The listing builds one solid part. Answer for the finished solid, in the listing's coordinates (mm). A direction names the side the tool comes from. Give positions to 0.01 mm unless a question says otherwise; leave off trailing zeros. Order: outer loops, then holes, each group sorted by start corner. A loop starts at its lowest first (then second) coordinate and runs counter-clockwise, first axis right, second up.
```python
from build123d import *

# Parameters (mm, degrees)
F1_DEPTH = 40
F2_R     = 5


with BuildPart() as f1:
    # F0 (on Front) → F1 (new body)
    with BuildSketch(Plane.XZ):
        Polygon((30, 0), (0, 0), (-20, 10), (-20, 30), (-30, 30), (-30, -10), (30, -10), align=None)
    extrude(amount=F1_DEPTH)

    # F2
    f2_edges = [f1.edges().sort_by_distance(p)[0] for p in [
        (30, -40, -5),
        (30, 0, -5),
        (-25, -40, 30),
        (-25, 0, 30),
    ]]
    fillet(f2_edges, radius=F2_R)


solid = f1.part
```
1) A tool of negligible diameter and unlimited length cuts with its end or side. For faces 1 (the flat face through (30, -20, -5)), 2 (the flat face through (15, -20, 0)), from which of +Z, -Z, +X, -X, +Y, -Y can it reach the whole face along a straight path? Write none if from no direction.
Geometry says:
face 1: +Z, -Z, +X, +Y, -Y
face 2: +Z, +X, +Y, -Y
2) Given P1, Ø3, axis at y = -6.5, z = 8, coming from the +X side; P2, Ø1, axis at y = -17.5, z = 24.5, coming from the +X side; P3, Ø9, axis at x = 14, y = -26.5, coming from the +Z side, each flat-ended and moving along its own axis, determine where each tip first touches the part or whether it passes through.
Geometry says:
P1: stops at x = -13
P2: stops at x = -20
P3: stops at z = 0
3) Find section B-B (x = -12). Write down the section's boundary in (y, z), then the cut area to 3 significant figures.
Geometry says:
outline: (-40, -10) - (0, -10) - (0, 6) - (-40, 6) - close
area: 640 mm2
4) Find section C-C (z = 6). Write down the section's boundary in (x, y), then the cut area to 3 significant figures.
Geometry says:
outline: (-30, -40) - (-12, -40) - (-12, 0) - (-30, 0) - close
area: 720 mm2
5) Straight lines are drawn through the part: probe 1 along X at (y, z) = (-7, 21); probe 2 along Z at (x, y) = (19, -3); probe 3 along Z at (x, y) = (-8.5, -15.5). For each, find the intervals that lie inside material, in ascending order.
Geometry says:
probe 1: x = -30 to -20
probe 2: z = -10 to 0
probe 3: z = -10 to 4.25
6) Find section A-A (y = -15.5). Write down the section's boundary in (x, z), then the cut area to 3 significant figures.
Geometry says:
outline: (-30, -10) - (30, -10) - (30, 0) - (0, 0) - (-20, 10) - (-20, 30) - (-30, 30) - close
area: 1,000 mm2
